The figure shows three views and two pictorial views of one solid part (mm, origin at its lowest corner). Answer the questions. Coordinates: 2 decimals unless noted, no trailing zeros. Order: outer loops, then holes, each group sorted by start corner. A loop starts at its lowest first (then second) coordinate and runs counter-clockwise, first axis right, second up. Notation, with made-up numbers: (-6, 85) -> (45, 85) arc R27 cw to (45, 111) -> close; hole circle Ø6 at (48.25, -28). An arc over 180 degrees is marked (long way). Use one line per item in the form item = value.
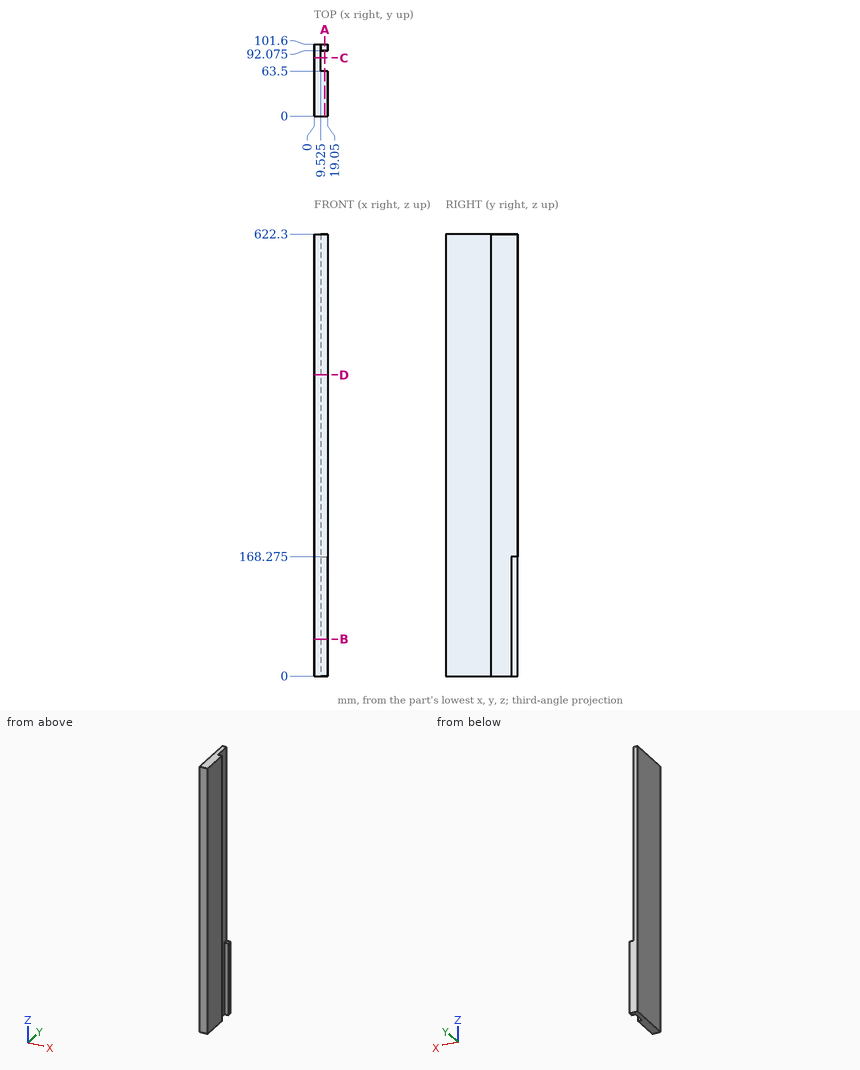
(1) Each of these flat-tipped pins is pushed along its axis until it touches: P1, Ø1, axis at x = 15, z = 206.5, coming from the +Y side; P2, Ø5, axis at x = 15.5, y = 95, coming from the +Z side (3 decimals); P3, Ø11.5, axis at y = 85.5, z = 202, coming from the +X side (3 decimals). Where does it stop, or does it pass through?
Data:
P1 = 63.5
P2 = 168.275
P3 = 9.525
(2) Section D-D on z = 424 is taken. Write down the section's boundary in (x, y) (3 decimals).
Data:
outline = (0, 0) -> (19.05, 0) -> (19.05, 63.5) -> (9.525, 63.5) -> (9.525, 101.6) -> (0, 101.6) -> close
(3) Section C-C on y = 82 is taken. Write down the section's boundary in (x, z) (3 decimals), plus the area to 3 significant figures.
Data:
outline = (0, 0) -> (9.525, 0) -> (9.525, 622.3) -> (0, 622.3) -> close
area = 5,930 mm²
(4) Section B-B on z = 52 is taken. Write down the section's boundary in (x, y) (3 decimals), plus the area to 3 significant figures.
Data:
outline = (0, 0) -> (19.05, 0) -> (19.05, 63.5) -> (9.525, 63.5) -> (9.525, 92.075) -> (19.05, 92.075) -> (19.05, 101.6) -> (0, 101.6) -> close
area = 1,660 mm²
(5) Section A-A on x = 15 is taken. Write down the section's boundary in (y, z) (3 decimals), plus the area to 3 significant figures.
Data:
outline = (0, 0) -> (63.5, 0) -> (63.5, 622.3) -> (0, 622.3) -> close; (92.075, 0) -> (101.6, 0) -> (101.6, 168.275) -> (92.075, 168.275) -> close
area = 41,100 mm²
(6) Straight lines are drawn through the part: line 1 along Y through (x, z) = (18.25, 68.5) (3 decimals); line 2 along Y through (x, z) = (15.75, 304); line 3 along X through (y, z) = (77, 188) (3 decimals). For each, find the intervals that lie inside material, in ascending order.
Data:
line_1 = 0 to 63.5, 92.075 to 101.6
line_2 = 0 to 63.5
line_3 = 0 to 9.525
